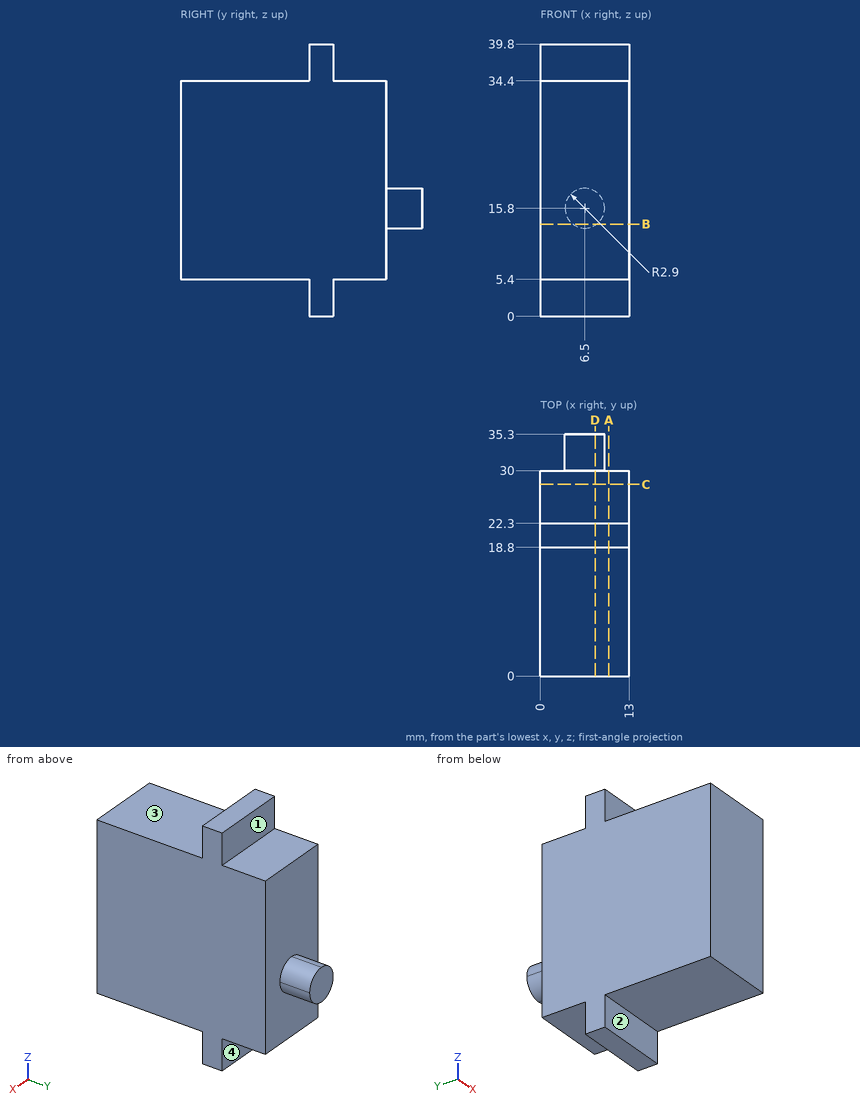
For this review, use the dimensioned drawing (mm, ordinates from the lowest corner) and the shaded views. A direction names the side the tool comes from. Round coordinates to 2 decimals unless told otherwise and drop trailing zeros. Order: outer loops, then holes, each group sorted by start corner. A loop starts at its lowest first (then second) coordinate and runs counter-clockwise, first axis right, second up.
1) Clearance check with flat-ended pins moving along their axes: pin 1 Ø4.5 at (x, z) = (9.5, 36) entering from +Y; pin 2 Ø4 at (x, y) = (4, 24.5) entering from +Z; pin 3 Ø2 at (x, y) = (2, 15) entering from -Z. State where each tip first meets the part, or that it passes through.
The answers:
pin 1: stops at y = 30
pin 2: stops at z = 34.4
pin 3: stops at z = 5.4
2) Consider section C-C (y = 28). State the section outline as (x, z) points, plus the area to 3 significant figures.
The answers:
outline: (0, 5.4) - (13, 5.4) - (13, 34.4) - (0, 34.4) - close
area: 377 mm2
3) Machinability: for the marked faces 1, 2, 3 and 4, which of the approach directions +Z, -Z, +X, -X, +Y, -Y give a long, thin tool a straight path to every point of the face, cutting with its end or side? Answer none if there is none.
The answers:
face 1: +Z, +X, -X, +Y
face 2: -Z, +X, -X, -Y
face 3: +Z, +X, -X, -Y
face 4: -Z, +X, -X, +Y
4) Consider section A-A (x = 10). State the section outline as (y, z) points.
The answers:
outline: (0, 5.4) - (18.8, 5.4) - (18.8, 0) - (22.3, 0) - (22.3, 5.4) - (30, 5.4) - (30, 34.4) - (22.3, 34.4) - (22.3, 39.8) - (18.8, 39.8) - (18.8, 34.4) - (0, 34.4) - close
5) Consider section D-D (x = 8). State the section outline as (y, z) points, plus the area to 3 significant figures.
The answers:
outline: (0, 5.4) - (18.8, 5.4) - (18.8, 0) - (22.3, 0) - (22.3, 5.4) - (30, 5.4) - (30, 13.32) - (35.3, 13.32) - (35.3, 18.28) - (30, 18.28) - (30, 34.4) - (22.3, 34.4) - (22.3, 39.8) - (18.8, 39.8) - (18.8, 34.4) - (0, 34.4) - close
area: 934 mm2
6) Consider section B-B (z = 13.5). State the section outline as (x, y) points.
The answers:
outline: (0, 0) - (13, 0) - (13, 30) - (8.27, 30) - (8.27, 35.3) - (4.73, 35.3) - (4.73, 30) - (0, 30) - close
7) For L1, parallel to Y at x = 7.25, z = 33.5; L2, parallel to Z at x = 7, y = 29.5; L3, parallel to Y at x = 1.5, z = 38.5, list the stretches that pass through material, from the lowest coordinate up.
The answers:
L1: y = 0 to 30
L2: z = 5.4 to 34.4
L3: y = 18.8 to 22.3
